For this review, take the finished solid that the model builds, in its own axes (mm). A direction names the side the tool comes from. Give positions to 0.01 mm unless a question says otherwise; leave off trailing zeros. Loops run counter-clockwise (first coordinate to the right, second up) from the corner with the lowest first, then second, coordinate; pieces in that order, holes last. Notation, with made-up numbers: (84, 58) - (138, 58) arc R18 cw to (138, 92) - close; hole circle Ø9 at (40.25, 55.25). An arc over 180 degrees is marked (long way). Put each result on its own line as item: value.
from build123d import *

# Parameters (mm, degrees)
F1_DEPTH  = 25.4
F2_R      = 5.08
F3_R      = 5.08
F4_W      = 41.3342826068
F4_H      = 24.7943252325
F5_DEPTH  = 25.4
F6_R      = 5.08
F7_T      = -2.54
F8_R      = 6.3689638983
F9_DEPTH  = 25.4
F10_R     = 6.6217822458
F11_DEPTH = 25


with BuildPart() as f1:
    # F0 (on Top) → F1 (new body)
    with BuildSketch(Plane.XY):
        Polygon((28.8636367768, 56.9190941751), (-58.8818192482, 56.9190941751), (-58.8818192482, -31.0572721064), (-19.8581814766, -31.0572721064), (-19.8581814766, -50.6845451891), (49.6454536915, -50.6845451891), (49.6454536915, 16.2790901959), (28.8636367768, 16.2790901959), align=None)
    extrude(amount=F1_DEPTH)

    # F2
    f2_edges = [f1.edges().sort_by_distance(p)[0] for p in [
        (14.893636, -50.684545, 25.4),
    ]]
    fillet(f2_edges, radius=F2_R)

    # F3
    f3_edges = [f1.edges().sort_by_distance(p)[0] for p in [
        (49.645454, -14.662727, 25.4),
    ]]
    fillet(f3_edges, radius=F3_R)

    # F4 (on face) → F5 (join)
    with BuildSketch(Plane.XY.offset(25.4)):
        with Locations((-5.3013917059, 12.3971626163)):
            Rectangle(F4_W, F4_H)
    extrude(amount=F5_DEPTH)

    # F6
    f6_edges = [f1.edges().sort_by_distance(p)[0] for p in [
        (15.36575, 0, 38.1),
    ]]
    fillet(f6_edges, radius=F6_R)

    # F7
    f7_openings = [f1.faces().sort_by_distance(p)[0] for p in [
        (-5.684641, 3.684325, 0),
    ]]
    offset(amount=F7_T, openings=f7_openings, kind=Kind.INTERSECTION)

    # F8 (on face) → F9 (join)
    with BuildSketch(Plane.XY.offset(50.8)):
        with Locations((-8.8408561423, 10.9183397144)):
            Circle(F8_R)
    extrude(amount=F9_DEPTH)

    # F10 (on face) → F11 (join)
    with BuildSketch(Plane.XY.offset(25.4)):
        with Locations((-41.423138231, 0)):
            Circle(F10_R)
    extrude(amount=F11_DEPTH)


solid = f1.part
1) Take a section at D-D on y = 44.5. State the section outline as (x, z) points, and give its area (3 significant figures).
Geometry check:
outline: (-58.88, 0) - (-56.34, 0) - (-56.34, 22.86) - (26.32, 22.86) - (26.32, 0) - (28.86, 0) - (28.86, 25.4) - (-58.88, 25.4) - close
area: 339 mm²
2) Take a section at B-B on y = -40. State the section outline as (x, z) points.
Geometry check:
outline: (-19.86, 0) - (-17.32, 0) - (-17.32, 22.86) - (44.57, 22.86) arc R2.54 cw to (47.11, 20.32) - (47.11, 0) - (49.65, 0) - (49.65, 20.32) arc R5.08 ccw to (44.57, 25.4) - (-19.86, 25.4) - close
3) Wall thickness on line 1 (Y direction, x = -22, z = 42.5); line 2 (X direction, y = 21, z = 22); line 3 (Y direction, x = -32.5, z = 10): over which ranges is each line inside the solid? List them lowest first.
Geometry check:
line 1: y = 0 to 2.54, 22.25 to 24.79
line 2: x = -58.88 to -56.34, 26.32 to 28.86
line 3: y = -31.06 to -28.52, 54.38 to 56.92
4) Insertion check: pin 1 Ø4 at (x, z) = (-26.5, 23) entering from -Y; pin 2 Ø12.5 at (x, z) = (-6, 37) entering from -Y; pin 3 Ø8 at (y, z) = (24, 19) entering from +X. Each pin has a flat end and moves straight along its axis. Give the tip position at first contact, or say it passes through.
Geometry check:
pin 1: stops at y = -31.06
pin 2: stops at y = 0
pin 3: stops at x = 28.86
5) Draft analysis for pull direction Y (two halves, no side actions). For faces 5 (the face through (-38.368, -5.875, 37.725)), 6 (the face through (-56.342, 14, 11)), 7 (the face through (49.645, -15, 10)), state which applies: pulls with the +Y half, pulls with the -Y half, needs draft (parallel to the pull), parting line crosses it, or undercut.
Geometry check:
face 5: parting line crosses it
face 6: undercut
face 7: needs draft
6) For faces 1 (the face through (15.366, 15, 38)), 2 (the face through (-6, 24.794, 38)), 3 (the face through (-6, 22.254, 35)), 4 (the face through (-10.22, 4.7, 63.32)), list the 3-axis set-ups (+Z, -Z, +X, -X, +Y, -Y) from which the entire face can be reached by the end or side of a thin tool; tool diameter is ignored.
Geometry check:
face 1: +Z, +X, +Y, -Y
face 2: +Z, +X, -X, +Y
face 3: -Z
face 4: +Z
7) Take a section at C-C on z = 12.5. State the section outline as (x, y) points, and give its area (3 significant figures).
Geometry check:
outline: (-58.88, -31.06) - (-19.86, -31.06) - (-19.86, -50.68) - (44.57, -50.68) arc R5.08 ccw to (49.65, -45.6) - (49.65, 16.28) - (28.86, 16.28) - (28.86, 56.92) - (-58.88, 56.92) - close; hole (-56.34, -28.52) - (-17.32, -28.52) - (-17.32, -48.14) - (44.57, -48.14) arc R2.54 ccw to (47.11, -45.6) - (47.11, 13.74) - (26.32, 13.74) - (26.32, 54.38) - (-56.34, 54.38) - close
area: 1,070 mm²
8) Take a section at A-A on x = 4. State the section outline as (y, z) points, and give its area (3 significant figures).
Geometry check:
outline: (-50.68, 0) - (-48.14, 0) - (-48.14, 20.32) arc R2.54 cw to (-45.6, 22.86) - (2.54, 22.86) - (2.54, 48.26) - (22.25, 48.26) - (22.25, 22.86) - (54.38, 22.86) - (54.38, 0) - (56.92, 0) - (56.92, 25.4) - (24.79, 25.4) - (24.79, 50.8) - (0, 50.8) - (0, 25.4) - (-45.6, 25.4) arc R5.08 ccw to (-50.68, 20.32) - close
area: 514 mm²
